Geometry: final body of the model. Coordinates: model frame, mm. Face numbers are marked on the shaded views. Round coordinates to 2 decimals unless told otherwise and drop trailing zeros. Loops run counter-clockwise (first coordinate to the right, second up) from the corner with the lowest first, then second, coordinate; pieces in that order, holes last. Notation, with made-up numbers: (-28, -33) -> (15, -33) arc R14 ccw to (15, -16) -> close; hole circle Ø6 at (-16, -33). An arc over 180 degrees is marked (long way). Answer in a Markdown table with one row per item.
```python
from build123d import *

# Parameters (mm, degrees)
SKETCH_1_R          = 16
EXTRUDE_1_DEPTH     = 10
SKETCH_2_R          = 12.5
SKETCH_2_R_2        = 10.25
EXTRUDE_2_DEPTH     = 30
SKETCH_3_R          = 2.1
CUT_EXTRUDE_1_DEPTH = 8
SKETCH_5_R          = 3.1
CUT_EXTRUDE_2_DEPTH = 15
CHAMFER_1_SIZE      = 3.5


with BuildPart() as part:
    # 草图1 → 凸台-拉伸1 (new body)
    with BuildSketch(Plane.XY):
        Circle(SKETCH_1_R)
    extrude(amount=EXTRUDE_1_DEPTH)

    # 草图2 → 凸台-拉伸2 (add)
    with BuildSketch(Plane(origin=(0, 0, 0), x_dir=(-1, 0, 0), z_dir=(0, 0, -1))):
        with Locations(Location((0, 0, 0), (0, 0, 180))):
            Circle(SKETCH_2_R)
        Circle(SKETCH_2_R_2, mode=Mode.SUBTRACT)
    extrude(amount=EXTRUDE_2_DEPTH)

    # 草图3 → 切除-拉伸1 (cut)
    with BuildSketch(Plane.XY.offset(10)):
        with Locations((-8.044168072, 8.044168072)):
            Circle(SKETCH_3_R)
        with Locations((8.044168072, 8.044168072)):
            Circle(SKETCH_3_R)
        with Locations((8.044168072, -8.044168072)):
            Circle(SKETCH_3_R)
        with Locations((-8.044168072, -8.044168072)):
            Circle(SKETCH_3_R)
    extrude(amount=-CUT_EXTRUDE_1_DEPTH, mode=Mode.SUBTRACT)

    # 草图5 → 切除-拉伸2 (cut, symmetric)
    with BuildSketch(Plane(origin=(0, 0, 0), x_dir=(1, 0, 0), z_dir=(0, 1, 0))):
        with Locations(Location((0, 20, 0), (0, 0, 270))):
            Circle(SKETCH_5_R)
    extrude(amount=CUT_EXTRUDE_2_DEPTH, both=True, mode=Mode.SUBTRACT)

    # 倒角1
    chamfer_1_edges = [part.edges().sort_by_distance(p)[0] for p in [
        (-12.5, 0, 0),
    ]]
    chamfer(chamfer_1_edges, length=CHAMFER_1_SIZE - 0.0001)  # a hair under: the kernel refuses the full size


solid = part.part
```
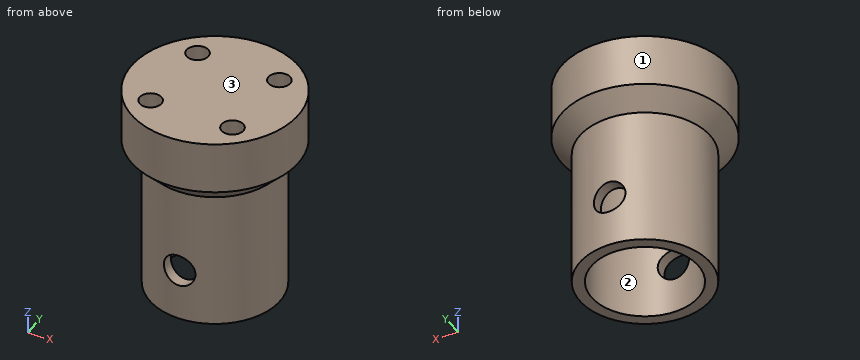
Item 1: Section query A-A, the plane x = 0. State how many separate pieces and enclosed holes the cut face has, and give its area (3 significant figures).
Ans:
| item | result |
|---|---|
| separate pieces | 3 |
| enclosed holes | 0 |
| area | 439 mm2 |
Item 2: Section query C-C, the plane z = -20. Output: boundary loops of the cut face in (x, y).
Ans:
| item | result |
|---|---|
| outline | (-3.1, -12.11) -> (-3.1, -9.77) arc R10.25 cw to (-3.1, 9.77) -> (-3.1, 12.11) arc R12.5 ccw to start; (3.1, -12.11) arc R12.5 ccw to (3.1, 12.11) -> (3.1, 9.77) arc R10.25 cw to (3.1, -9.77) -> close |
Item 3: Mould query, pull axis Y, two halves, no side actions, for the marked faces 1, 2 and 3. Classes: released by +Y, released by -Y, zero draft, split by the parting line, or undercut.
Ans:
| item | result |
|---|---|
| face 1 | split by the parting line |
| face 2 | undercut |
| face 3 | zero draft |
Item 4: First-contact query: P1, Ø2.5, axis at x = 8.04, y = -8.04, coming from the +Z side; P2, Ø1.5, axis at x = -11, z = -19.5, coming from the +Y side; P3, Ø1, axis at x = 12, z = -18, coming from the +Y side. Flat tips, straight axial feed; report the tip coordinate or a pass-through.
Ans:
| item | result |
|---|---|
| P1 | z = 2 |
| P2 | y = 7.15 |
| P3 | y = 4.9 |
Item 5: Ray query, L1, parallel to Z at x = 0, y = 11; L2, parallel to Y at x = 0, z = -14.5; L3, parallel to Z at x = -10, y = 0. Return the intervals inside material, ascending.
Ans:
| item | result |
|---|---|
| L1 | -30 to -23.1, -16.9 to 10 |
| L2 | -12.5 to -10.25, 10.25 to 12.5 |
| L3 | 0 to 10 |
Item 6: Section query D-D, the plane z = -12. Output: boundary loops of the cut face in (x, y).
Ans:
| item | result |
|---|---|
| outline | circle Ø25 at (0, 0); hole circle Ø20.5 at (0, 0) |
